```python
from build123d import *

# Parameters (mm, degrees)
SKETCH002_R     = 2.2
SKETCH002_R_2   = 1.45
PAD002_DEPTH    = 15.5
SKETCH003_R     = 33
SKETCH003_R_2   = 2.2
PAD003_DEPTH    = 4.5
POCKET_DEPTH    = 3
POCKET001_DEPTH = 4
POCKET003_DEPTH = 2
SKETCH011_W     = 5.5
SKETCH011_H     = 11.1
POCKET004_DEPTH = 25.001
SKETCH012_W     = 3.4
SKETCH012_H     = 17.1165875376
PAD007_DEPTH    = 7.75
POCKET005_DEPTH = 229.0145930205
SKETCH017_R     = 0.75
POCKET008_DEPTH = 17.1165875376
PAD008_DEPTH    = 5
SKETCH020_R     = 0.6
POCKET009_DEPTH = 3.0152762344
FILLET_R        = 3
CHAMFER_SIZE    = 4
CHAMFER001_SIZE = 4
FILLET006_R     = 2
FILLET007_R     = 2


with BuildPart() as part:
    # Sketch002 (on Face1 of ShapeBinder) → Pad002 (new body)
    with BuildSketch(Plane.XZ.offset(37.5)):
        with BuildLine():
            Line((-32.0156211872, -8), (32.0156211872, -8))
            ThreePointArc((26.9599822671, -19.0304849165), (29.9991391555, -13.7496054463), (32.0156211872, -8))
            Line((-26.9599822671, -19.0304849165), (26.9599822671, -19.0304849165))
            ThreePointArc((-32.0156211872, -8), (-29.9991391555, -13.7496054463), (-26.9599822671, -19.0304849165))
        make_face()
        with Locations((24, -11)):
            Circle(SKETCH002_R, mode=Mode.SUBTRACT)
        with Locations((0, -11)):
            Circle(SKETCH002_R_2, mode=Mode.SUBTRACT)
        with Locations((-24, -11)):
            Circle(SKETCH002_R, mode=Mode.SUBTRACT)
    extrude(amount=PAD002_DEPTH)

    # Sketch003 (on Face9 of Pad002) → Pad003 (join)
    with BuildSketch(Plane.XZ.offset(53)):
        Circle(SKETCH003_R)
        with Locations((24, -11)):
            Circle(SKETCH003_R_2, mode=Mode.SUBTRACT)
        with Locations((-24, -11)):
            Circle(SKETCH003_R_2, mode=Mode.SUBTRACT)
    extrude(amount=PAD003_DEPTH)

    # Sketch007 (on Face2 of Pad003) → Pocket (cut)
    with BuildSketch(Plane(origin=(0, -4.5, -8), x_dir=(1, 0, 0), z_dir=(0, 0, 1))):
        with BuildLine():
            ThreePointArc((1.45, -35), (0, -33.55), (-1.45, -35))
            Line((-1.45, -35), (-1.45, -45))
            Line((-1.45, -45), (1.45, -45))
            Line((1.45, -35), (1.45, -45))
        make_face()
    extrude(amount=-POCKET_DEPTH, mode=Mode.SUBTRACT)

    # Sketch008 (on Face16 of Pocket) → Pocket001 (cut)
    with BuildSketch(Plane.XZ.offset(57.5)):
        Polygon((27.7, -13.136195996), (27.7, -8.863804004), (24, -6.727608008), (20.3, -8.863804004), (20.3, -13.136195996), (24, -15.272391992), align=None)
        Polygon((-20.3, -13.136195996), (-20.3, -8.863804004), (-24, -6.727608008), (-27.7, -8.863804004), (-27.7, -13.136195996), (-24, -15.272391992), align=None)
    extrude(amount=-POCKET001_DEPTH, mode=Mode.SUBTRACT)

    # Sketch010 (on Face10 of Pocket001) → Pocket003 (cut)
    with BuildSketch(Plane(origin=(0, -49.5, 0), x_dir=(-1, 0, 0), z_dir=(0, 1, 0))):
        with BuildLine():
            ThreePointArc((-11, -11.0000000007), (6e-10, -22), (11, -10.9999999995))
            Line((11, 0), (11, -10.9999999995))
            Line((-11, 0), (11, 0))
            Line((-11, 0), (-11, -11.0000000007))
        make_face()
    extrude(amount=-POCKET003_DEPTH, mode=Mode.SUBTRACT)

    # Sketch011 (on Face2 of Pocket003) → Pocket004 (cut, through all)
    with BuildSketch(Plane(origin=(0, -4.5, -8), x_dir=(1, 0, 0), z_dir=(0, 0, 1))):
        with Locations((17.2656211872, -40.75)):
            Rectangle(SKETCH011_W, SKETCH011_H)
    extrude(amount=-POCKET004_DEPTH, mode=Mode.SUBTRACT)

    # Sketch012 (on Face6 of Pocket004) → Pad007 (join)
    with BuildSketch(Plane(origin=(0, -53, 0), x_dir=(-1, 0, 0), z_dir=(0, 1, 0))):
        with Locations((-3.4, 23.2352590367)):
            Rectangle(SKETCH012_W, SKETCH012_H)
        with Locations((3.4, 23.2352590367)):
            Rectangle(SKETCH012_W, SKETCH012_H)
    extrude(amount=PAD007_DEPTH)

    # Sketch013 (on Face33 of Pad007) → Pocket005 (cut, through all)
    with BuildSketch(Plane(origin=(5.1, -4.5, 0), x_dir=(0, 1, 0), z_dir=(1, 0, 0))):
        with BuildLine():
            ThreePointArc((-42.925, 28.7693325629), (-44.625, 30.4693325629), (-46.325, 28.7693325629))
            Line((-46.325, 28.7693325629), (-46.325, 17.7011855106))
            ThreePointArc((-46.325, 17.7011855106), (-44.625, 16.0011855106), (-42.925, 17.7011855106))
            Line((-42.925, 28.7693325629), (-42.925, 17.7011855106))
        make_face()
    extrude(amount=-POCKET005_DEPTH, mode=Mode.SUBTRACT)

    # Sketch017 (on Face30 of Pocket005) → Pocket008 (cut)
    with BuildSketch(Plane(origin=(0, -4.5, 31.7935528056), x_dir=(1, 0, 0), z_dir=(0, 0, 1))):
        with Locations((-3.3679491924, -41.75)):
            Circle(SKETCH017_R)
        with Locations((3.3679491924, -41.75)):
            Circle(SKETCH017_R)
        with Locations((-3.3679491924, -47.5)):
            Circle(SKETCH017_R)
        with Locations((3.3679491924, -47.5)):
            Circle(SKETCH017_R)
    extrude(amount=-POCKET008_DEPTH, mode=Mode.SUBTRACT)

    # Sketch019 (on Face6 of Pocket008) → Pad008 (join)
    with BuildSketch(Plane(origin=(0, -53, 0), x_dir=(-1, 0, 0), z_dir=(0, 1, 0))):
        with BuildLine():
            ThreePointArc((29.3729634054, 15.0409115677), (28.645422971, 16.3841308226), (27.8564999708, 17.6922415023))
            Line((25.3564999708, 17.6922415023), (27.8564999708, 17.6922415023))
            Line((25.3564999708, 17.6922415023), (25.3564999708, 14.6769652679))
            Line((25.3564999708, 14.6769652679), (29.1504409553, 14.6769652679))
            ThreePointArc((29.1504409553, 14.6769652679), (29.3637325104, 14.796555481), (29.3729634054, 15.0409115677))
        make_face()
    pad008 = extrude(amount=PAD008_DEPTH)

    # Sketch020 (on Face30 of Pad008) → Pocket009 (cut)
    with BuildSketch(Plane(origin=(0, -4.5, 17.6922415023), x_dir=(1, 0, 0), z_dir=(0, 0, 1))):
        with Locations((-26.988867595, -45.2352647517)):
            Circle(SKETCH020_R)
        with Locations((-26.2241323467, -46.7647352483)):
            Circle(SKETCH020_R)
    pocket009 = extrude(amount=-POCKET009_DEPTH, mode=Mode.SUBTRACT)

    # Mirrored: Pad008 across Sketch019 V_Axis
    add(pad008.mirror(Plane(origin=(0, -53, 0), x_dir=(0, 1, 0), z_dir=(-1, 0, 0))))

    # Mirrored001: Pocket009 across Sketch020 V_Axis
    add(pocket009.mirror(Plane(origin=(0, -4.5, 17.6922415023), x_dir=(0, 0, 1), z_dir=(1, 0, 0))), mode=Mode.SUBTRACT)

    # Fillet
    fillet_edges = [part.edges().sort_by_distance(p)[0] for p in [
        (5.1, -53, 23.235259),
        (-5.1, -53, 23.235259),
    ]]
    fillet(fillet_edges, radius=FILLET_R)

    # Chamfer
    chamfer_edges = [part.edges().sort_by_distance(p)[0] for p in [
        (-25.3565, -53, 16.184603),
    ]]
    chamfer(chamfer_edges, length=CHAMFER_SIZE)

    # Chamfer001
    chamfer001_edges = [part.edges().sort_by_distance(p)[0] for p in [
        (25.3565, -53, 16.184603),
    ]]
    chamfer(chamfer001_edges, length=CHAMFER001_SIZE)

    # Fillet006
    fillet006_edges = [part.edges().sort_by_distance(p)[0] for p in [
        (-25.3565, -49, 16.184603),
    ]]
    fillet(fillet006_edges, radius=FILLET006_R)

    # Fillet007
    fillet007_edges = [part.edges().sort_by_distance(p)[0] for p in [
        (25.3565, -49, 16.184603),
    ]]
    fillet(fillet007_edges, radius=FILLET007_R)


solid = part.part
```
Geometry check sheet. Reference: the model listing, model coordinates, mm. A direction names the side the tool comes from. Coordinates: 2 decimals unless noted, no trailing zeros. Write each loop counter-clockwise with the first axis right and the second up, starting at its lowest first coordinate (ties: lowest second). Pieces come first, ordered by that corner, then holes. Notation, with made-up numbers: (74.25, 27.5) -> (82.25, 27.5) arc R22 ccw to (82.25, 56.5) -> close; hole circle Ø5 at (53.5, 27.5). An arc over 180 degrees is marked (long way). Use CSV: the item, a comma, the result in double quotes. Start each with the question number.
Item 1: Cross-section at D-D, the plane x = -10. Record the cut outline in (y, z), plus the area to 3 significant figures.
Item 2: Cross-section at A-A, the plane x = 23. Record the cut outline in (y, z), plus the area to 3 significant figures.
Item 3: Cross-section at C-C, the plane z = 26.5. State how many separate pieces and enclosed holes the cut face has, plus the area to 3 significant figures.
Item 4: Thickness scan on line 1 (Y direction, x = 3.5, z = 21) (3 decimals); line 2 (Y direction, x = 3, z = -8.5); line 3 (Z direction, x = -24.5, y = -40.5). Record the ranges inside material, lowest first.
Item 5: Mould release check, pull along X, two halves, no side actions. Record for faces 4 (the flat face through (-22.18, -55.53, -14.22)), 5 (the flat face through (-3, -50.825, 23)): released by +X, released by -X, zero draft, split by the parting line, or undercut.
Item 6: Depth check by flat-ended pin: pin 1 Ø7 at (x, z) = (-24, -11) entering from -Y; pin 2 Ø10 at (x, y) = (-6, -54.5) entering from -Z; pin 3 Ø4 at (x, y) = (17.5, -53) entering from +Z; pin 4 Ø12 at (x, z) = (-25.5, -9) entering from -Y. Enter the tip coordinate at first touch or a pass-through.
Item 7: Cross-section at B-B, the plane z = 0. Record the cut outline in (x, y).
Item 8: Set-up check for faces 1 (the flat face through (0, -53, -24)), 2 (the flat face through (23.088, -51.269, 16.206)), 3 (the cylindrical face through (3.27, -45.506, 23.355)): record each of +Z, -Z, +X, -X, +Y, -Y from which the full face is reachable in a straight line by a thin tool's end or side.
Answers:
1,outline,"(-57.5, -31.45) -> (-53, -31.45) -> (-53, -19.03) -> (-37.5, -19.03) -> (-37.5, -8) -> (-49.5, -8) -> (-49.5, -15.58) -> (-51.5, -15.58) -> (-51.5, -8) -> (-53, -8) -> (-53, 31.45) -> (-57.5, 31.45) -> close"
1,area,"439 mm^2"
2,outline,"(-57.5, -23.66) -> (-53, -23.66) -> (-53, -19.03) -> (-37.5, -19.03) -> (-37.5, -12.96) -> (-53.5, -12.96) -> (-53.5, -14.7) -> (-57.5, -14.7) -> close; (-57.5, -7.3) -> (-53.5, -7.3) -> (-53.5, -9.04) -> (-37.5, -9.04) -> (-37.5, -8) -> (-53, -8) -> (-53, 14.68) -> (-51.36, 14.68) -> (-51.36, 17.69) -> (-53, 17.69) -> (-53, 23.66) -> (-57.5, 23.66) -> close"
2,area,"297 mm^2"
3,separate pieces,"3"
3,enclosed holes,"4"
3,area,"203 mm^2"
4,line 1,"-57.5 to -52.738, -51.262 to -50.825, -47.425 to -46.988, -45.512 to -45.25"
4,line 2,"-57.5 to -51.5, -49.5 to -37.5"
4,line 3,"-19.03 to -13.14, -8.86 to -8"
5,face 4,"undercut"
5,face 5,"zero draft"
6,pin 1,"y = -53.5"
6,pin 2,"z = -32.98"
6,pin 3,"z = 29.13"
6,pin 4,"y = -57.5"
7,outline,"(-33, -57.5) -> (33, -57.5) -> (33, -53) -> (-33, -53) -> close"
8,face 1,"-Z, +X, -X, +Y"
8,face 2,"+Z, +Y"
8,face 3,"+Z"
